```python
from build123d import *

# Parameters (mm, degrees)
F1_DEPTH = 19
F2_R     = 14
F2_R_2   = 10
F3_DEPTH = 17
F4_R     = 18.99999
F5_R     = 10
F6_DEPTH = 8.001
F7_W     = 8
F7_H     = 18
F8_DEPTH = 38


# Not quite as in the source:
# - a fillet or chamfer is up to 0.001 mm smaller than in the source, because OpenCascade refuses the exact size


with BuildPart() as f1:
    # F0 (on Front) → F1 (new body, symmetric)
    with BuildSketch(Plane.XZ):
        Polygon((0, 68), (0, 0), (73, 0), (73, 8), (8, 8), (8, 68), align=None)
    extrude(amount=F1_DEPTH, both=True)

    # F2 (on face) → F3 (join)
    with BuildSketch(Plane.YZ.offset(8)):
        with Locations((2.5166787673, 50)):
            Circle(F2_R)
        with Locations((2.5166787673, 50)):
            Circle(F2_R_2, mode=Mode.SUBTRACT)
    extrude(amount=F3_DEPTH)

    # F4 (radius 19 in the source; OpenCascade refuses exactly that, so slightly less here)
    f4_edges = [f1.edges().sort_by_distance(p)[0] for p in [
        (73, -19, 4),
        (73, 19, 4),
    ]]
    fillet(f4_edges, radius=F4_R)

    # F5 (on face) → F6 (cut, through all)
    with BuildSketch(Plane.XY.offset(8)):
        with Locations((54, 0)):
            Circle(F5_R)
    extrude(amount=-F6_DEPTH, mode=Mode.SUBTRACT)

    # F7 (on face) → F8 (join, through all)
    with BuildSketch(Plane.XZ.offset(19)):
        with Locations((32, 17)):
            Rectangle(F7_W, F7_H)
    extrude(amount=-F8_DEPTH)


solid = f1.part
```
Read the model definition and answer for the solid it produces. Units are mm, in the model's axes. A direction names the side the tool comes from. Coordinates: 2 decimals unless noted, no trailing zeros. Loops run counter-clockwise (first coordinate to the right, second up) from the corner with the lowest first, then second, coordinate; pieces in that order, holes last. Notation, with made-up numbers: (3, -16) -> (55, -16) arc R15 cw to (55, 0) -> close; hole circle Ø5 at (-14.5, -19.5). An arc over 180 degrees is marked (long way). Return JSON: item names as keys, results as strings.
Item 1: For a pull along Z with two mould halves and no side action, classify faces 1 (the flat face through (4, 0, 68)), 2 (the cylindrical face through (16.381, 0.349, 40.238)), 3 (the cylindrical face through (67.29, 13.58, 4.06)) as +Z half, -Z half, draft (parallel to the pull), parting line (faces both ways), or undercut.
Answers:
{"face 1": "+Z half", "face 2": "undercut", "face 3": "draft"}
Item 2: For faces 4 (the flat face through (28, 0, 17)), 5 (the flat face through (25, -1, 60)), 6 (the cylindrical face through (16.381, -0.518, 36.333)), determine the directions among +Z, -Z, +X, -X, +Y, -Y from which every point of the face is accessible in a straight line to the end or side of a thin tool.
Answers:
{"face 4": "+Z, +Y, -Y", "face 5": "+Z, +X, +Y, -Y", "face 6": "+X"}
Item 3: Flat-ended cylindrical pins translate along their axes: P1, Ø10, axis at y = 0, z = 48.5, coming from the +X side; P2, Ø3, axis at x = 35.5, y = 8, coming from the +Z side; P3, Ø16, axis at x = 21, y = 0, coming from the +Z side. Find the tip coordinate at first contact, or state that the pin passes through.
Answers:
{"P1": "stops at x = 8", "P2": "stops at z = 26", "P3": "stops at z = 64"}
Item 4: Find section C-C (z = 50). Determine the outline of the cut face in (x, y).
Answers:
{"outline": "(0, -19) -> (8, -19) -> (8, -11.48) -> (25, -11.48) -> (25, -7.48) -> (8, -7.48) -> (8, 12.52) -> (25, 12.52) -> (25, 16.52) -> (8, 16.52) -> (8, 19) -> (0, 19) -> close"}
Item 5: Find section B-B (y = -3.5). Determine the outline of the cut face in (x, z).
Answers:
{"outline": "(0, 0) -> (44.63, 0) -> (44.63, 8) -> (36, 8) -> (36, 26) -> (28, 26) -> (28, 8) -> (8, 8) -> (8, 37.36) -> (25, 37.36) -> (25, 42.01) -> (8, 42.01) -> (8, 57.99) -> (25, 57.99) -> (25, 62.64) -> (8, 62.64) -> (8, 68) -> (0, 68) -> close; (63.37, 0) -> (72.67, 0) -> (72.67, 8) -> (63.37, 8) -> close"}
Item 6: Find section D-D (x = 34). Determine the outline of the cut face in (y, z), plus the area to 3 significant figures.
Answers:
{"outline": "(-19, 0) -> (19, 0) -> (19, 26) -> (-19, 26) -> close", "area": "988 mm2"}
Item 7: Find the intervals of material crossed by probe 1 along X at (y, z) = (-15, 18); probe 2 along X at (y, z) = (13.5, 34), in increasing order.
Answers:
{"probe 1": "x = 0 to 8, 28 to 36", "probe 2": "x = 0 to 8"}
